from build123d import *

# Parameters (mm, degrees)
F0_R       = 35
F1_DEPTH   = 1
F2_W       = 1
F2_H       = 1
F3_DEPTH   = 15
F4_R       = 29
F5_DEPTH   = 16.001
F6_SIZE2   = 10
F6_SIZE    = 1.5
F7_SIZE2   = 2.5
F7_SIZE    = 10
F7_2_SIZE2 = 2.5
F7_2_SIZE  = 10
F7_3_SIZE2 = 2.5
F7_3_SIZE  = 10
F7_4_SIZE2 = 2.5
F7_4_SIZE  = 10
F7_5_SIZE2 = 2.5
F7_5_SIZE  = 10
F7_6_SIZE2 = 2.5
F7_6_SIZE  = 10
F7_7_SIZE2 = 2.5
F7_7_SIZE  = 10
F7_8_SIZE2 = 2.5
F7_8_SIZE  = 10


with BuildPart() as f1:
    # F0 (on Top) → F1 (new body)
    with BuildSketch(Plane.XY):
        Circle(F0_R)
    extrude(amount=F1_DEPTH)

    # F2 (on face) → F3 (join)
    with BuildSketch(Plane.XY.offset(1)):
        with BuildLine():
            Line((31, 0), (32, 0))
            ThreePointArc((32, 0), (29.7519001173, 11.7823783426), (23.323472537, 21.9092589746))
            Line((23.323472537, 21.9092589746), (22.627416998, 21.2132034356))
            Line((22.627416998, 21.2132034356), (21.9203102168, 21.9203102168))
            Line((21.9203102168, 21.9203102168), (22.627416998, 22.627416998))
            ThreePointArc((22.627416998, 22.627416998), (12.7063707016, 29.3691699507), (1, 31.9843711834))
            Line((1, 31.9843711834), (1, 31))
            Line((1, 31), (0, 31))
            Line((0, 31), (0, 32))
            ThreePointArc((0, 32), (-11.7823783426, 29.7519001173), (-21.9092589746, 23.323472537))
            Line((-21.9092589746, 23.323472537), (-21.2132034356, 22.627416998))
            Line((-21.2132034356, 22.627416998), (-21.9203102168, 21.9203102168))
            Line((-21.9203102168, 21.9203102168), (-22.627416998, 22.627416998))
            ThreePointArc((-22.627416998, 22.627416998), (-29.3691699507, 12.7063707016), (-31.9843711834, 1))
            Line((-31.9843711834, 1), (-31, 1))
            Line((-31, 1), (-31, 0))
            Line((-31, 0), (-32, 0))
            ThreePointArc((-32, 0), (-29.7519001173, -11.7823783426), (-23.323472537, -21.9092589746))
            Line((-23.323472537, -21.9092589746), (-22.627416998, -21.2132034356))
            Line((-22.627416998, -21.2132034356), (-21.9203102168, -21.9203102168))
            Line((-21.9203102168, -21.9203102168), (-22.627416998, -22.627416998))
            ThreePointArc((-22.627416998, -22.627416998), (-12.7063707016, -29.3691699507), (-1, -31.9843711834))
            Line((-1, -31.9843711834), (-1, -31))
            Line((-1, -31), (0, -31))
            Line((0, -31), (0, -32))
            ThreePointArc((0, -32), (11.7823783426, -29.7519001173), (21.9092589746, -23.323472537))
            Line((21.9092589746, -23.323472537), (21.2132034356, -22.627416998))
            Line((21.2132034356, -22.627416998), (21.9203102168, -21.9203102168))
            Line((21.9203102168, -21.9203102168), (22.627416998, -22.627416998))
            ThreePointArc((22.627416998, -22.627416998), (29.3691699507, -12.7063707016), (31.9843711834, -1))
            Line((31.9843711834, -1), (31, -1))
            Line((31, -1), (31, 0))
        make_face()
        with BuildLine():
            Line((32, -1), (32, 0))
            ThreePointArc((32, 0), (31.9960925573, -0.5000610612), (31.9843711834, -1))
            Line((31.9843711834, -1), (32, -1))
        make_face()
        with BuildLine():
            ThreePointArc((31.9843711834, -1), (31.9960925573, -0.5000610612), (32, 0))
            Line((32, 0), (31, 0))
            Line((31, 0), (31, -1))
            Line((31, -1), (31.9843711834, -1))
        make_face()
        with Locations((32.5, -0.5)):
            Rectangle(F2_W, F2_H)
        with BuildLine():
            Line((22.627416998, 21.2132034356), (23.323472537, 21.9092589746))
            ThreePointArc((23.323472537, 21.9092589746), (22.9782505862, 22.2710574513), (22.627416998, 22.627416998))
            Line((22.627416998, 22.627416998), (21.9203102168, 21.9203102168))
            Line((21.9203102168, 21.9203102168), (22.627416998, 21.2132034356))
        make_face()
        with BuildLine():
            ThreePointArc((22.627416998, 22.627416998), (22.9782505862, 22.2710574513), (23.323472537, 21.9092589746))
            Line((23.323472537, 21.9092589746), (23.3345237792, 21.9203102168))
            Line((23.3345237792, 21.9203102168), (22.627416998, 22.627416998))
        make_face()
        Polygon((23.3345237792, 23.3345237792), (22.627416998, 22.627416998), (23.3345237792, 21.9203102168), (24.0416305603, 22.627416998), align=None)
        with BuildLine():
            Line((21.9203102168, -23.3345237792), (22.627416998, -22.627416998))
            ThreePointArc((22.627416998, -22.627416998), (22.2710574513, -22.9782505862), (21.9092589746, -23.323472537))
            Line((21.9092589746, -23.323472537), (21.9203102168, -23.3345237792))
        make_face()
        with BuildLine():
            ThreePointArc((21.9092589746, -23.323472537), (22.2710574513, -22.9782505862), (22.627416998, -22.627416998))
            Line((22.627416998, -22.627416998), (21.9203102168, -21.9203102168))
            Line((21.9203102168, -21.9203102168), (21.2132034356, -22.627416998))
            Line((21.2132034356, -22.627416998), (21.9092589746, -23.323472537))
        make_face()
        Polygon((23.3345237792, -23.3345237792), (22.627416998, -22.627416998), (21.9203102168, -23.3345237792), (22.627416998, -24.0416305603), align=None)
        with BuildLine():
            Line((1, 31), (1, 31.9843711834))
            ThreePointArc((1, 31.9843711834), (0.5000610612, 31.9960925573), (0, 32))
            Line((0, 32), (0, 31))
            Line((0, 31), (1, 31))
        make_face()
        with BuildLine():
            ThreePointArc((0, 32), (0.5000610612, 31.9960925573), (1, 31.9843711834))
            Line((1, 31.9843711834), (1, 32))
            Line((1, 32), (0, 32))
        make_face()
        with Locations((0.5, 32.5)):
            Rectangle(F2_W, F2_H)
        with BuildLine():
            Line((-1, -32), (0, -32))
            ThreePointArc((0, -32), (-0.5000610612, -31.9960925573), (-1, -31.9843711834))
            Line((-1, -31.9843711834), (-1, -32))
        make_face()
        with BuildLine():
            ThreePointArc((-1, -31.9843711834), (-0.5000610612, -31.9960925573), (0, -32))
            Line((0, -32), (0, -31))
            Line((0, -31), (-1, -31))
            Line((-1, -31), (-1, -31.9843711834))
        make_face()
        with Locations((-0.5, -32.5)):
            Rectangle(F2_W, F2_H)
        with BuildLine():
            Line((-21.2132034356, 22.627416998), (-21.9092589746, 23.323472537))
            ThreePointArc((-21.9092589746, 23.323472537), (-22.2710574513, 22.9782505862), (-22.627416998, 22.627416998))
            Line((-22.627416998, 22.627416998), (-21.9203102168, 21.9203102168))
            Line((-21.9203102168, 21.9203102168), (-21.2132034356, 22.627416998))
        make_face()
        with BuildLine():
            ThreePointArc((-22.627416998, 22.627416998), (-22.2710574513, 22.9782505862), (-21.9092589746, 23.323472537))
            Line((-21.9092589746, 23.323472537), (-21.9203102168, 23.3345237792))
            Line((-21.9203102168, 23.3345237792), (-22.627416998, 22.627416998))
        make_face()
        Polygon((-23.3345237792, 23.3345237792), (-22.627416998, 22.627416998), (-21.9203102168, 23.3345237792), (-22.627416998, 24.0416305603), align=None)
        with BuildLine():
            Line((-23.3345237792, -21.9203102168), (-22.627416998, -22.627416998))
            ThreePointArc((-22.627416998, -22.627416998), (-22.9782505862, -22.2710574513), (-23.323472537, -21.9092589746))
            Line((-23.323472537, -21.9092589746), (-23.3345237792, -21.9203102168))
        make_face()
        with BuildLine():
            ThreePointArc((-23.323472537, -21.9092589746), (-22.9782505862, -22.2710574513), (-22.627416998, -22.627416998))
            Line((-22.627416998, -22.627416998), (-21.9203102168, -21.9203102168))
            Line((-21.9203102168, -21.9203102168), (-22.627416998, -21.2132034356))
            Line((-22.627416998, -21.2132034356), (-23.323472537, -21.9092589746))
        make_face()
        Polygon((-23.3345237792, -23.3345237792), (-22.627416998, -22.627416998), (-23.3345237792, -21.9203102168), (-24.0416305603, -22.627416998), align=None)
        with BuildLine():
            Line((-31, 1), (-31.9843711834, 1))
            ThreePointArc((-31.9843711834, 1), (-31.9960925573, 0.5000610612), (-32, 0))
            Line((-32, 0), (-31, 0))
            Line((-31, 0), (-31, 1))
        make_face()
        with BuildLine():
            ThreePointArc((-32, 0), (-31.9960925573, 0.5000610612), (-31.9843711834, 1))
            Line((-31.9843711834, 1), (-32, 1))
            Line((-32, 1), (-32, 0))
        make_face()
        with Locations((-32.5, 0.5)):
            Rectangle(F2_W, F2_H)
    extrude(amount=F3_DEPTH)

    # F4 (on face) → F5 (cut, through all)
    with BuildSketch(Plane.XY.offset(16)):
        Circle(F4_R)
    extrude(amount=-F5_DEPTH, mode=Mode.SUBTRACT)

    # F6
    f6_edges = [f1.edges().sort_by_distance(p)[0] for p in [
        (12.706371, 29.36917, 16),
        (29.7519, 11.782378, 16),
        (29.36917, -12.706371, 16),
        (11.782378, -29.7519, 16),
        (-12.706371, -29.36917, 16),
        (-29.7519, -11.782378, 16),
        (-29.36917, 12.706371, 16),
        (-11.782378, 29.7519, 16),
    ]]
    f6_side = f1.faces().sort_by_distance((28.512525, -12.335749, 16))[0]
    chamfer(f6_edges, length=F6_SIZE, length2=F6_SIZE2, reference=f6_side)

    # F7
    f7_edges = [f1.edges().sort_by_distance(p)[0] for p in [
        (33, -0.5, 16),
    ]]
    f7_side = f1.faces().sort_by_distance((33, -0.5, 8.5))[0]
    chamfer(f7_edges, length=F7_SIZE, length2=F7_SIZE2, reference=f7_side)

    # F7#2
    f7_2_edges = [f1.edges().sort_by_distance(p)[0] for p in [
        (22.98097, -23.688077, 16),
    ]]
    f7_2_side = f1.faces().sort_by_distance((22.98097, -23.688077, 8.5))[0]
    chamfer(f7_2_edges, length=F7_2_SIZE, length2=F7_2_SIZE2, reference=f7_2_side)

    # F7#3
    f7_3_edges = [f1.edges().sort_by_distance(p)[0] for p in [
        (-0.5, -33, 16),
    ]]
    f7_3_side = f1.faces().sort_by_distance((-0.5, -33, 8.5))[0]
    chamfer(f7_3_edges, length=F7_3_SIZE, length2=F7_3_SIZE2, reference=f7_3_side)

    # F7#4
    f7_4_edges = [f1.edges().sort_by_distance(p)[0] for p in [
        (-23.688077, -22.98097, 16),
    ]]
    f7_4_side = f1.faces().sort_by_distance((-23.688077, -22.98097, 8.5))[0]
    chamfer(f7_4_edges, length=F7_4_SIZE, length2=F7_4_SIZE2, reference=f7_4_side)

    # F7#5
    f7_5_edges = [f1.edges().sort_by_distance(p)[0] for p in [
        (-33, 0.5, 16),
    ]]
    f7_5_side = f1.faces().sort_by_distance((-33, 0.5, 8.5))[0]
    chamfer(f7_5_edges, length=F7_5_SIZE, length2=F7_5_SIZE2, reference=f7_5_side)

    # F7#6
    f7_6_edges = [f1.edges().sort_by_distance(p)[0] for p in [
        (-22.98097, 23.688077, 16),
    ]]
    f7_6_side = f1.faces().sort_by_distance((-22.98097, 23.688077, 8.5))[0]
    chamfer(f7_6_edges, length=F7_6_SIZE, length2=F7_6_SIZE2, reference=f7_6_side)

    # F7#7
    f7_7_edges = [f1.edges().sort_by_distance(p)[0] for p in [
        (0.5, 33, 16),
    ]]
    f7_7_side = f1.faces().sort_by_distance((0.5, 33, 8.5))[0]
    chamfer(f7_7_edges, length=F7_7_SIZE, length2=F7_7_SIZE2, reference=f7_7_side)

    # F7#8
    f7_8_edges = [f1.edges().sort_by_distance(p)[0] for p in [
        (23.688077, 22.98097, 16),
    ]]
    f7_8_side = f1.faces().sort_by_distance((23.688077, 22.98097, 8.5))[0]
    chamfer(f7_8_edges, length=F7_8_SIZE, length2=F7_8_SIZE2, reference=f7_8_side)


solid = f1.part
Design review of the part built by this model. Coordinates are the model's own, in mm. A direction names the side the tool comes from. Round coordinates to 2 decimals unless told otherwise and drop trailing zeros. Use one line per item in the form item = value. Start each with the question number.
Q1. Wall thickness on line 1 along Z through (x, y) = (29, 19); line 2 along Y through (x, z) = (-3, 14.75); line 3 along X through (y, z) = (7.5, 15): over which ranges is each line inside the solid? List them lowest first. Write a range as [from, to].
Q2. For pin 1 Ø5 at (x, z) = (-14.5, 12) entering from -Y; pin 2 Ø4 at (y, z) = (6.5, 12) entering from -X; pin 3 Ø0.8 at (x, z) = (0.5, 3.5) entering from +Y, all flat-tipped, find the tip position at first contact; note any pin that passes through.
Q3. Machinability: for faces 1 (the face through (-0.507, -31.732, 11.07)), 2 (the face through (32.3, 0, 6.2)), which of the approach directions +Z, -Z, +X, -X, +Y, -Y give a long, thin tool a straight path to every point of the face, cutting with its end or side? Answer none if there is none.
Q4. Draft analysis for pull direction Y (two halves, no side actions). For faces 3 (the face through (11.357, -29.125, 10.93)), 4 (the face through (13.38, -25.73, 8.11)), 5 (the face through (23, -23, 6)), 6 (the face through (0.493, 31.732, 11.07)), state which applies: +Y half, -Y half, draft (parallel to the pull), parting line (faces both ways), or undercut.
Calculated:
q1.line_1 = [0, 1]
q1.line_2 = [-30.54, -28.84], [28.84, 30.54]
q1.line_3 = [-29.72, -28.01], [28.01, 29.72]
q2.pin_1 = -28.77
q2.pin_2 = -30.9
q2.pin_3 = 33
q3.face_1 = +Z, +X, -X, -Y
q3.face_2 = +Z, +X, +Y
q4.face_3 = -Y half
q4.face_4 = undercut
q4.face_5 = undercut
q4.face_6 = +Y half
